```python
from build123d import *

# Parameters (mm, degrees)
F0_R     = 25.4
F1_DEPTH = 6.35
F4_SIZE  = 1.27
F9_R     = 1.5875


with BuildPart() as f1:
    # F0 (on Top) → F1 (new body)
    with BuildSketch(Plane.XY):
        Circle(F0_R)
    extrude(amount=-F1_DEPTH)

    # F2 (on Front) → F3 (revolve)
    with BuildSketch(Plane.XZ):
        Polygon((19.85, -6.35), (0, -6.35), (0, -31.75), (9.525, -31.75), (9.525, -16.2), (22.225, -16.2), (22.225, -9.85), (19.85, -9.85), align=None)
    revolve(axis=Axis((0, 0, -19.05), (0, 0, 1)))

    # F4
    f4_edges = [f1.edges().sort_by_distance(p)[0] for p in [
        (-22.225, 0, -9.85),
        (-22.225, 0, -16.2),
    ]]
    chamfer(f4_edges, length=F4_SIZE)

    # F5 (on Front) → F6 (revolve, cut)
    with BuildSketch(Plane.XZ):
        Polygon((20.32, 0), (0, 0), (0, -6.35), (10.8669128953, -6.35), (12.7, -3.175), (20.32, -3.175), align=None)
        Polygon((10.8669128953, -6.35), (0, -6.35), (0, -42.1200841665), (6.35, -42.1200841665), (6.35, -14.1735226281), align=None)
    revolve(axis=Axis((0, 0, 5.083523225), (0, 0, 1)), mode=Mode.SUBTRACT)

    # F7 (on Front) → F8 (revolve, cut)
    with BuildSketch(Plane.XZ):
        Polygon((16.51, -31.75), (16.51, -16.2), (9.525, -16.2), (8.89, -16.2), (8.89, -31.75), (9.525, -31.75), align=None)
        Polygon((9.525, -16.2), (16.51, -16.2), (16.51, -6.675), (13.6122134253, -6.675), (8.89, -14.8541135768), (8.89, -16.2), align=None)
    revolve(axis=Axis((0, 0, -10.6237775408), (0, 0, 1)), mode=Mode.SUBTRACT)

    # F9
    f9_edges = [f1.edges().sort_by_distance(p)[0] for p in [
        (-16.51, 0, -6.675),
        (16.51, 0, -11.4375),
        (-13.612213, 0, -6.675),
        (-20.32, 0, -3.175),
        (-8.89, 0, -14.854114),
    ]]
    fillet(f9_edges, radius=F9_R)


solid = f1.part
```
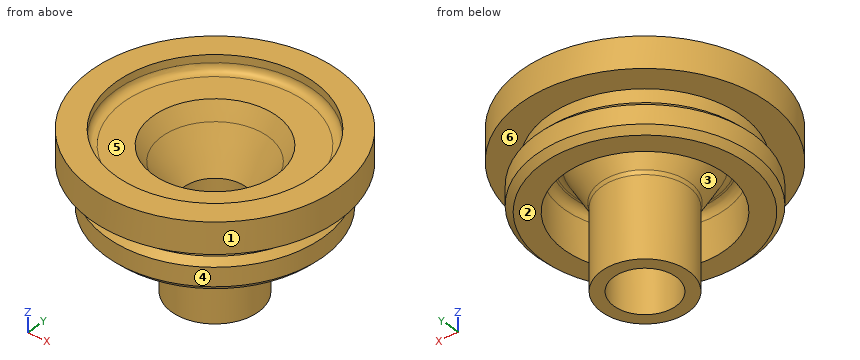
Model file for the job. Use its own axes, mm. Face numbers are marked on the shaded views. A direction names the side the tool comes from. Coordinates: 2 decimals unless noted, no trailing zeros. Write each loop counter-clockwise with the first axis right and the second up, starting at its lowest first coordinate (ties: lowest second). Pieces come first, ordered by that corner, then holes. Notation, with made-up numbers: (-30.5, 17.25) - (18.5, 17.25) arc R26 ccw to (18.5, 48.25) - close; hole circle Ø8 at (13.25, -38). An arc over 180 degrees is marked (long way). Use a Markdown table: item, result. Add a question column.
Item 1: Band-saw the part on A-A, the plane z = -19.5. Write the cut outline in (x, y), and give its area (3 significant figures).
Item 2: Two-plate mould, pull along Y, no slides. Class the marked faces 1, 2 and 3: pulls with the +Y half, pulls with the -Y half, needs draft (parallel to the pull), parting line crosses it, or undercut.
Item 3: 3-axis set-ups, long thin cutter, end or side, ignore diameter. For the marked faces 4, 5 and 6: which of +Z, -Z, +X, -X, +Y, -Y reach the whole face in a straight line?
Item 4: Drill centre lines: line 1 along Y through (x, z) = (5.5, -15); line 2 along Y through (x, z) = (0, -20); line 3 along Z through (x, y) = (-16, 13). Where is each one in solid material? Low to high.
Item 5: Drop flat-ended pins along their axis: pin 1 (18.5 mm diameter, centred on x = -5.5, y = -3, fed in from +Z) (3 decimals); pin 2 (5 mm diameter, centred on x = -8, z = -8.5, fed in from +Y); pin 3 (1.5 mm diameter, centred on x = 2, y = 18, fed in from -Z). Give the stop position or say it passes through.
A:
| question | item | result |
|---|---|---|
| 1 | outline | circle Ø17.78 at (0, 0); hole circle Ø12.7 at (0, 0) |
| 1 | area | 122 mm² |
| 2 | face 1 | parting line crosses it |
| 2 | face 2 | needs draft |
| 2 | face 3 | undercut |
| 3 | face 4 | -Z |
| 3 | face 5 | +Z |
| 3 | face 6 | none |
| 4 | line 1 | y = -21.46 to -15.57, -7.02 to -3.17, 3.17 to 7.02, 15.57 to 21.46 |
| 4 | line 2 | y = -8.89 to -6.35, 6.35 to 8.89 |
| 4 | line 3 | z = -16.2 to -9.85, -6.35 to 0 |
| 5 | pin 1 | stops at z = -3.175 |
| 5 | pin 2 | stops at y = 24.49 |
| 5 | pin 3 | stops at z = -16.2 |
